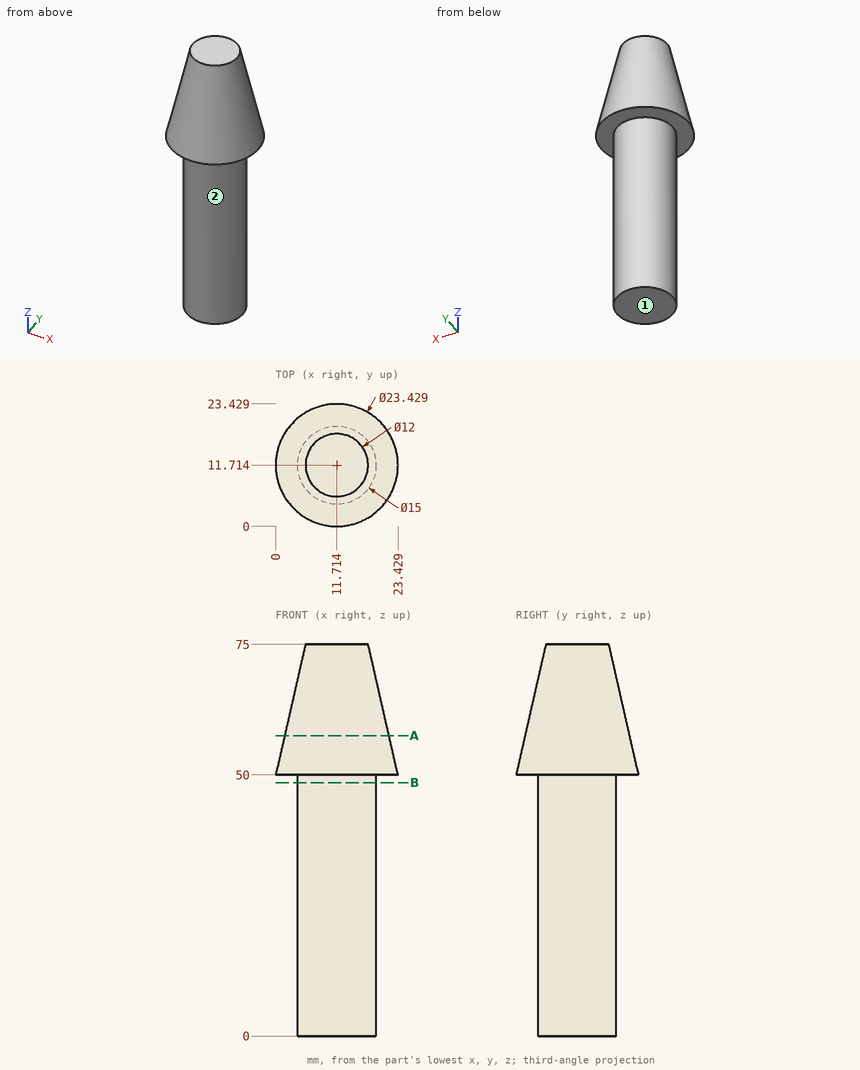
Study the drawing (mm; zero at the part's minimum x, y, z) and answer. A direction names the side the tool comes from. Round coordinates to 2 decimals unless told otherwise and drop trailing zeros. Order: outer loops, then holes, each group sorted by start corner. A loop starts at its lowest first (then second) coordinate and runs counter-clockwise, first axis right, second up. Notation, with made-up numbers: (-25, 58.25) -> (14, 58.25) arc R32 ccw to (14, 85.25) -> close; hole circle Ø11 at (9, 82). An arc over 180 degrees is marked (long way). Write each question's results on one line, items separated by ' | '. Start each with the question number.
Q1. Which of the six approach directions +Z, -Z, +X, -X, +Y, -Y give full straight-line access (tool end or side, diameter ignored) to the marked faces 1 and 2?
Q2. Straight lines are drawn through the part: probe 1 along Y at (x, z) = (13, 10) (1 decimal); probe 2 along Y at (x, z) = (16, 13); probe 3 along X at (y, z) = (20.5, 57.5) (1 decimal). For each, find the intervals that lie inside material, in ascending order. Write a range as from..to.
Q3. Find section A-A (z = 57.5). Determine the outline of the cut face in (x, y) (1 decimal), then the cut area to 3 significant figures.
Q4. Each of these flat-tipped pins is pushed along its axis until it touches: pin 1 (12 mm diameter, centred on x = 13.5, z = 65, fed in from -Y); pin 2 (4 mm diameter, centred on y = 3.5, z = 66.5, fed in from -X); pin 3 (8 mm diameter, centred on y = 10, z = 25.5, fed in from +X); pin 4 (8 mm diameter, centred on x = 8, y = 10, fed in from -Z). Where does it stop, or does it pass through?
Q5. Find section B-B (z = 48.5). Determine the outline of the cut face in (x, y) (1 decimal).
Worked answers:
1) face 1: -Z, +X, -X, +Y, -Y | face 2: -Z
2) probe 1: y = 4.3..19.1 | probe 2: y = 5.56..17.87 | probe 3: x = 6.9..16.5
3) outline: circle Ø20 at (11.7, 11.7) | area: 314 mm2
4) pin 1: stops at y = 2.1 | pin 2: stops at x = 6.66 | pin 3: stops at x = 19.21 | pin 4: stops at z = 0
5) outline: circle Ø15 at (11.7, 11.7)
